Input: part model. Units: mm. Frame: model coordinates. A direction names the side the tool comes from. Give positions to 0.01 mm unless a question says otherwise; leave off trailing zeros. Order: outer loops, then holes, each group sorted by start corner. A loop starts at its lowest first (then second) coordinate and runs counter-clockwise, first axis right, second up.
```python
from build123d import *

# Parameters (mm, degrees)
F0_W      = 7.9375
F0_H      = 15.875
F0_R      = 2.38125
F1_DEPTH  = 9.525
F2_DEPTH  = 11.1125
F3_W      = 3.175
F3_H      = 2.38125
F4_DEPTH  = 3.175
F5_W      = 1.5875
F5_H      = 6.35
F6_DEPTH  = 6.35
F7_DEPTH  = 1.5875
F8_R      = 1.5875
F9_DEPTH  = 0.79375
F10_R     = 1.5875
F11_DEPTH = 0.79375


with BuildPart() as f1:
    # F0 (on Top) → F1 (new body)
    with BuildSketch(Plane.XY):
        Rectangle(F0_W, F0_H)
        with Locations((0, -3.96875)):
            Circle(F0_R, mode=Mode.SUBTRACT)
        with Locations((0, 3.96875)):
            Circle(F0_R, mode=Mode.SUBTRACT)
    extrude(amount=F1_DEPTH)

    # F0 (on Top) → F2 (join)
    with BuildSketch(Plane.XY):
        with Locations((0, 3.96875)):
            Circle(F0_R)
        with Locations((0, -3.96875)):
            Circle(F0_R)
    extrude(amount=F2_DEPTH)

    # F3 (on Right) → F4 (join, symmetric)
    with BuildSketch(Plane.YZ):
        with Locations((-9.525, 6.746875)):
            Rectangle(F3_W, F3_H)
        with Locations((-9.525, 4.365625)):
            Rectangle(F3_W, F3_H)
        with BuildLine():
            Line((-13.49375, 5.55625), (-11.1125, 5.55625))
            Line((-11.1125, 5.55625), (-11.1125, 7.9375))
            ThreePointArc((-11.1125, 7.9375), (-12.796298, 7.240048), (-13.49375, 5.55625))
        make_face()
        with BuildLine():
            Line((-11.1125, 3.175), (-11.1125, 5.55625))
            Line((-11.1125, 5.55625), (-13.49375, 5.55625))
            ThreePointArc((-13.49375, 5.55625), (-12.796298, 3.872452), (-11.1125, 3.175))
        make_face()
    extrude(amount=F4_DEPTH, both=True)

    # F5 (on face) → F6 (cut)
    with BuildSketch(Plane.XY.offset(7.9375)):
        with Locations((0.79375, -11.1125)):
            Rectangle(F5_W, F5_H)
        with Locations((-0.79375, -11.1125)):
            Rectangle(F5_W, F5_H)
    extrude(amount=-F6_DEPTH, mode=Mode.SUBTRACT)

    # F3 (on Right) → F7 (join, symmetric)
    with BuildSketch(Plane.YZ):
        Polygon((7.9375, 8.73125), (7.9375, 5.55625), (14.2875, 5.55625), (14.2875, 7.9375), align=None)
        Polygon((14.2875, 5.55625), (7.9375, 5.55625), (7.9375, 2.38125), (14.2875, 3.175), align=None)
    extrude(amount=F7_DEPTH, both=True)

    # F8 (on face) → F9 (cut)
    with BuildSketch(Plane.YZ.offset(1.5875)):
        with Locations((11.1125, 5.55625)):
            Circle(F8_R)
    extrude(amount=-F9_DEPTH, mode=Mode.SUBTRACT)

    # F10 (on face) → F11 (cut)
    with BuildSketch(Plane(origin=(-1.5875, 0, 0), x_dir=(0, -1, 0), z_dir=(-1, 0, 0))):
        with Locations((-11.1125, 5.55625)):
            Circle(F10_R)
    extrude(amount=-F11_DEPTH, mode=Mode.SUBTRACT)


solid = f1.part
```
1) First-contact query: P1, Ø1.9, axis at y = 12, z = 5, coming from the +X side; P2, Ø2.5, axis at x = 2, z = 4.5, coming from the +Y side; P3, Ø4, axis at y = -10, z = 6, coming from the -X side (3 decimals); P4, Ø1.7, axis at x = 2.5, y = -9.5, coming from the +Z side. Flat tips, straight axial feed; report the tip coordinate or a pass-through.
2) Cut plane B-B (z = 10.25). Return the cut outline in (x, y).
3) Cut plane D-D (y = 11.5). Return the cut outline in (x, z).
4) Line query: probe 1 along X at (y, z) = (-11.25, 7) (1 decimal); probe 2 along Y at (x, z) = (3.75, 5.5); probe 3 along Z at (x, y) = (3.5, -1.25) (3 decimals). Output: solid intervals per line, ascending.
5) Pull-direction query (Y, two-part tool) for faces 1 (the face through (0.02, 11.16, 8.33)), 2 (the face through (1.588, 10, 7)), 3 (the face through (-0.516, -6.293, 10.308)); classes: pulls with the +Y half, pulls with the -Y half, needs draft (parallel to the pull), parting line crosses it, or undercut.
6) Reachability of faces 4 (the face through (2, -10, 7.938)), 5 (the face through (-0.31, 6.33, 10.31)), 6 (the face through (-3.175, -11, 6)), 7 (the face through (-0.794, 11, 6)), 8 (the face through (3.175, -11, 6)) from +Z, -Z, +X, -X, +Y, -Y: full face, straight path, thin tool, end or side. Return the list, or none.
7) Cut plane A-A (y = -9.75). Return the cut outline in (x, z) (1 decimal).
Geometry says:
1. P1: stops at x = 1.59
1. P2: stops at y = 14.29
1. P3: stops at x = -3.175
1. P4: stops at z = 7.94
2. outline: circle Ø4.76 at (0, -3.97); circle Ø4.76 at (0, 3.97)
3. outline: (-1.59, 2.83) - (1.59, 2.83) - (1.59, 4.02) - (0.79, 4.02) - (0.79, 7.1) - (1.59, 7.1) - (1.59, 8.29) - (-1.59, 8.29) - (-1.59, 7.1) - (-0.79, 7.1) - (-0.79, 4.02) - (-1.59, 4.02) - close
4. probe 1: x = -3.2 to -1.6, 1.6 to 3.2
4. probe 2: y = -7.94 to 7.94
4. probe 3: z = 0 to 9.525
5. face 1: pulls with the +Y half
5. face 2: needs draft
5. face 3: undercut
6. face 4: +Z, +X, -X, -Y
6. face 5: +Z
6. face 6: +Z, -Z, -X, -Y
6. face 7: -X
6. face 8: +Z, -Z, +X, -Y
7. outline: (-3.2, 3.2) - (-1.6, 3.2) - (-1.6, 7.9) - (-3.2, 7.9) - close; (1.6, 3.2) - (3.2, 3.2) - (3.2, 7.9) - (1.6, 7.9) - close
